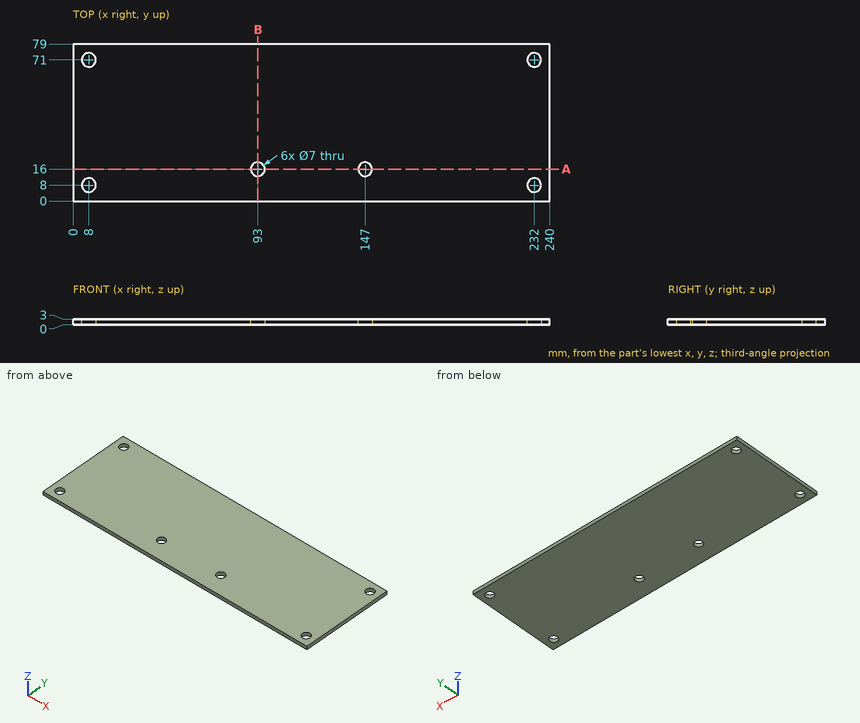
Print and shaded views of the part. All mm, measured from the part's lowest x, y and z. Round coordinates to 2 decimals unless told otherwise and drop trailing zeros. Write each loop counter-clockwise with the first axis right and the second up, starting at its lowest first coordinate (ties: lowest second). Pieces come first, ordered by that corner, then holes. Notation, with made-up numbers: (29, -7.75) -> (78, -7.75) arc R37 cw to (78, 31.25) -> close; hole circle Ø6 at (-35, 15). An arc over 180 degrees is marked (long way). Return JSON: item names as keys, results as strings. Group by question number.
Q1. Pin check, flat tip, straight feed: pin 1 (4 mm diameter, centred on x = 232, y = 71, fed in from +Z). Stop position of the tip, or through.
Q2. Saw through at B-B on x = 93. Write the cut outline in (y, z).
Q3. Saw through at A-A on y = 16. Write the cut outline in (x, z), plus the area to 3 significant figures.
Q4. Probe L1, parallel to Y at x = 8, z = 1.05; L2, parallel to Y at x = 93, z = 1.5; L3, parallel to Y at x = 229, z = 0.25. List the from-to ranges inside material, lowest first. Write a range as [from, to].
Answer:
{
 "1": {"pin 1": "through"},
 "2": {"outline": "(0, 0) -> (12.5, 0) -> (12.5, 3) -> (0, 3) -> close; (19.5, 0) -> (79, 0) -> (79, 3) -> (19.5, 3) -> close"},
 "3": {"outline": "(0, 0) -> (89.5, 0) -> (89.5, 3) -> (0, 3) -> close; (96.5, 0) -> (143.5, 0) -> (143.5, 3) -> (96.5, 3) -> close; (150.5, 0) -> (240, 0) -> (240, 3) -> (150.5, 3) -> close", "area": "678 mm2"},
 "4": {"L1": "[0, 4.5], [11.5, 67.5], [74.5, 79]", "L2": "[0, 12.5], [19.5, 79]", "L3": "[0, 6.2], [9.8, 69.2], [72.8, 79]"}
}
